The model under review builds one solid part; all positions refer to its coordinate system, in mm. A direction names the side the tool comes from. Coordinates: 2 decimals unless noted, no trailing zeros. Loops run counter-clockwise (first coordinate to the right, second up) from the corner with the lowest first, then second, coordinate; pieces in that order, holes last. Notation, with made-up numbers: M -18.5,41.25 L 34.5,41.25 A24 cw 34.5,78.25 Z; hole C 59,-37.5 d3. An arc over 180 degrees is marked long. Return JSON: item names as keys, results as strings.
Autodesk Inventor part; units mm, degrees
ref_plane "YZ Plane" through (0, 0, 0) normal (1, 0, 0) x (0, 1, 0)
ref_plane "XZ Plane" through (0, 0, 0) normal (0, 1, 0) x (-1, 0, 0)
ref_plane "XY Plane" through (0, 0, 0) normal (0, 0, 1) x (1, 0, 0)
sketch "Sketch1" plane through (0, 0, 0) normal (0, 0, 1) x (1, 0, 0)
  arc A0 (6.35, -145.9119) -> (0, 146.05) centre (0, 0) ccw
  line L0 (0, 0) -> (0, 323.4187) construction
  line L1 (0, 0) -> (0, -168.91) construction
  line L2 (6.35, -168.7906) -> (6.35, -145.9119)
  line L3 (6.35, 145.9119) -> (6.35, 168.7906)
  line L4 (0, -146.05) -> (0, -151.13)
  line L5 (0, -151.13) -> (6.35, -151.13)
  line L6 (6.35, -151.13) -> (-7.62, -151.13)
  line L7 (-7.62, -151.13) -> (-7.62, -161.29)
  line L8 (-7.62, -161.29) -> (6.35, -161.29)
  line L9 (0, 146.05) -> (0, 151.13)
  line L10 (0, 151.13) -> (6.35, 151.13)
  line L11 (6.35, 151.13) -> (-7.62, 151.13)
  line L12 (-7.62, 151.13) -> (-7.62, 161.29)
  line L13 (-7.62, 161.29) -> (6.35, 161.29)
  line L14 (168.91, 0) -> (168.91, -114.3)
  line L15 (168.91, -114.3) -> (124.3628, -114.3)
  arc A1 (124.3628, 114.3) -> (6.35, 168.7906) centre (0, 0) ccw
  arc A2 (6.35, -168.7906) -> (124.3628, -114.3) centre (0, 0) ccw
  line L16 (0, 0) -> (-12.7, 0)
  line L17 (-12.7, 0) -> (324.8812, 0) construction
  line L18 (168.91, 0) -> (168.91, 114.3)
  line L19 (168.91, 114.3) -> (124.3628, 114.3)
  line L20 (146.05, 0) -> (146.05, 82.55) construction
  line L21 (146.05, 82.55) -> (120.4828, 82.55) construction
  line L22 (146.05, 0) -> (146.05, -82.55) construction
  line L23 (146.05, -82.55) -> (120.4828, -82.55) construction
  line L24 (146.05, -82.55) -> (120.4828, -82.55) construction
  line L25 (130.6254, -90.1931) -> (121.4538, -102.3643)
  line L26 (121.4538, -102.3643) -> (104.1737, -102.3643)
  line L27 (130.6254, 90.1931) -> (121.447, 102.3733)
  line L28 (104.1648, 102.3733) -> (121.447, 102.3733)
  line L29 (130.6254, 90.1931) -> (130.6254, 65.3268)
  line L30 (130.6254, -90.1931) -> (130.6254, -65.3268)
  dimension "d0" = 292.1
  dimension "d7" = 6.35
  dimension "d8" = 6.35
  dimension "d9" = 5.08
  dimension "d10" = 13.97
  dimension "d11" = 10.16
  dimension "d12" = 5.08
  dimension "d13" = 13.97
  dimension "d14" = 10.16
  dimension "d16" = 5.2181
  dimension "d35" = 12.7
  dimension "d38" = 114.3
  dimension "d57" = 114.3
  dimension "d58" = 82.55
  dimension "d59" = 82.55
  dimension "d60" = 12.7
  dimension "d63" = 12.7
  dimension "d66" = 127
extrude "Extrusion2" add sketch "Sketch1" along normal blind 6.35 contours A0 L26 L25 L30 L29 L27 L28 L3 A1 L19 L18 L14 L15 A2 L2 | L2 L8 L7 L6 L5 | L10 L11 L12 L13 L3
sketch "Sketch3" plane through (0, 0, 6.35) normal (0, 0, 1) x (1, 0, 0)
  line L0 (124.3628, -114.3) -> (168.91, -114.3)
  line L1 (168.91, -114.3) -> (168.91, 114.3)
  line L2 (168.91, -114.3) -> (168.91, -43.2308) construction
  line L3 (168.91, -43.2308) -> (163.83, -43.2308) construction
  line L4 (163.83, -43.2308) -> (153.67, -43.2308)
  line L5 (153.67, -43.2308) -> (153.67, -33.7058)
  line L6 (153.67, -33.7058) -> (163.83, -33.7058)
  line L7 (163.83, -33.7058) -> (163.83, -43.2308)
  line L8 (168.91, -50.8) -> (149.86, -50.8)
  line L9 (149.86, -50.8) -> (149.86, -76.2)
  line L10 (149.86, -76.2) -> (149.86, -114.3)
  line L11 (149.86, -114.3) -> (168.91, -114.3)
  line L12 (168.91, -50.8) -> (168.91, -114.3)
  line L13 (168.91, -27.0751) -> (151.13, -27.0751)
  line L14 (151.13, -27.0751) -> (168.91, 0)
  line L15 (168.91, 0) -> (168.91, -27.0751)
  dimension "d46" = 71.0692
  dimension "d47" = 5.08
  dimension "d48" = 10.16
  dimension "d49" = 9.525
  dimension "d50" = 10.16
  dimension "d51" = 19.05
  dimension "d52" = 63.5
  dimension "d53" = 25.4
  dimension "d54" = 17.78
extrude "Extrusion5" cut sketch "Sketch3" against normal blind 25.4
properties part number "BottomHoop_v1" material "Polycarbonate, Clear"
1. To check wall thickness, follow line 1 (Y direction, x = 91.5, z = 3.75); line 2 (Y direction, x = 72, z = 2); line 3 (X direction, y = -36, z = 5). State the ranges of each line that lie inside material, in increasing order.
Check values:
{"line 1": "-141.98 to -113.83, 113.83 to 141.98", "line 2": "-152.8 to -127.07, 127.07 to 152.8", "line 3": "141.54 to 153.67, 163.83 to 168.91"}
2. Add section C-C on x = 77. Give the boundary of the cut face in (y, z), plus the area to 3 significant figures.
Check values:
{"outline": "M -150.34,0 L -124.1,0 L -124.1,6.35 L -150.34,6.35 Z; M 124.1,0 L 150.34,0 L 150.34,6.35 L 124.1,6.35 Z", "area": "333 mm²"}
3. Insertion check: pin 1 Ø3 at (x, z) = (148, 2.5) entering from +Y; pin 2 Ø2 at (y, z) = (-64.5, 4) entering from -X; pin 3 Ø3 at (x, z) = (27.5, 4.5) entering from -Y. Each pin has a flat end and moves straight along its axis. Give the tip position at first contact, or say it passes through.
Check values:
{"pin 1": "y = 114.3", "pin 2": "x = 130.63", "pin 3": "y = -166.9"}
4. The part is to be moulded in two halves that separate along Y. For faces 1 (the face through (-1, 161.29, 3)), 2 (the face through (160, -50.8, 3)), 3 (the face through (159, -33.706, 3)), say which applies: released by +Y, released by -Y, zero draft, split by the parting line, or undercut.
Check values:
{"face 1": "released by +Y", "face 2": "released by -Y", "face 3": "undercut"}
5. Machinability: for faces 4 (the face through (149.86, -82, 3)), 5 (the face through (6.35, -165, 3)), 6 (the face through (-1, -151.13, 3)), which of the approach directions +Z, -Z, +X, -X, +Y, -Y give a long, thin tool a straight path to every point of the face, cutting with its end or side? Answer none if there is none.
Check values:
{"face 4": "+Z, -Z, +X, -Y", "face 5": "+Z, -Z, -X, -Y", "face 6": "+Z, -Z, -X"}
6. Add section D-D on y = -107. Give the boundary of the cut face in (x, z).
Check values:
{"outline": "M 99.41,0 L 149.86,0 L 149.86,6.35 L 99.41,6.35 Z"}
7. Add section A-A on x = 116. Give the boundary of the cut face in (y, z), plus the area to 3 significant figures.
Check values:
{"outline": "M -122.78,0 L -102.36,0 L -102.36,6.35 L -122.78,6.35 Z; M 102.37,0 L 122.78,0 L 122.78,6.35 L 102.37,6.35 Z", "area": "259 mm²"}
